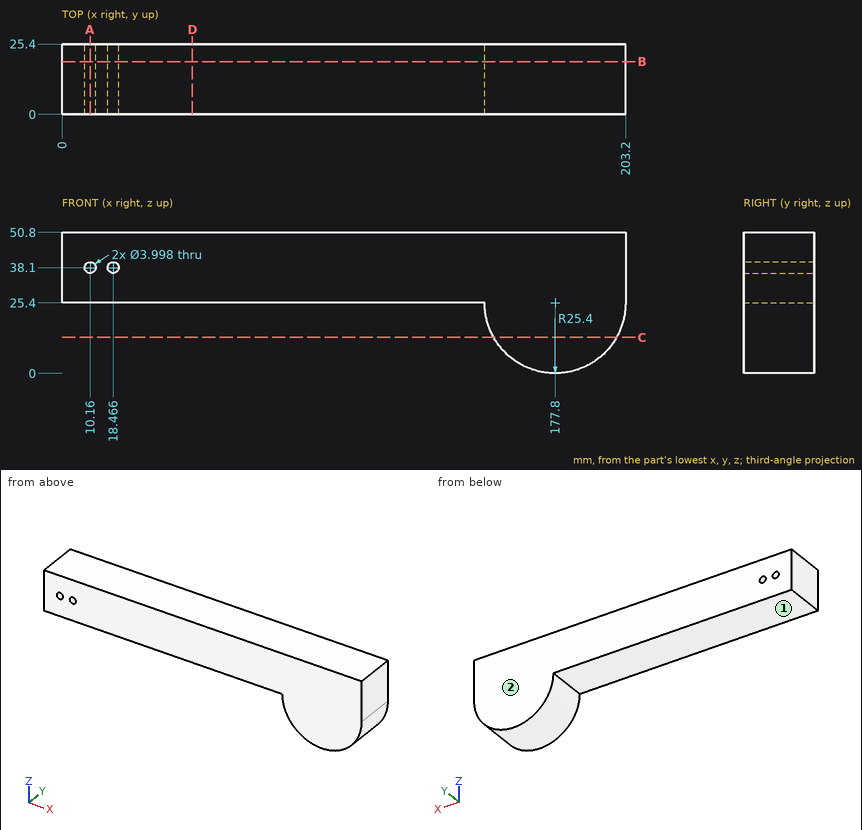
Study the drawing (mm; zero at the part's minimum x, y, z) and answer. A direction names the side the tool comes from. Give positions to 0.01 mm unless a question says otherwise; leave off trailing zeros. Write each loop counter-clockwise with the first axis right and the second up, starting at its lowest first coordinate (ties: lowest second). Pieces come first, ordered by that corner, then holes. Notation, with made-up numbers: (-34.5, -19) - (0.5, -19) arc R20 ccw to (0.5, -9) - close; hole circle Ø3 at (74.5, -16.5). An arc over 180 degrees is marked (long way). One line per question, with ' | ' between items. Start each with the question number.
1. Section D-D, the plane x = 47 is taken. Determine the outline of the cut face in (y, z).
2. Given P1, Ø1, axis at y = 6.5, z = 12.5, coming from the -X side; P2, Ø1, axis at y = 14.5, z = 23.5, coming from the -X side, each flat-ended and moving along its own axis, determine where each tip first touches the part or whether it passes through.
3. Straight lines are drawn through the part: line 1 (X direction, y = 20.25, z = 38.1) (1 decimal); line 2 (X direction, y = 16.25, z = 37) (1 decimal); line 3 (Z direction, x = 45.5, y = 2.25). For each, find the intervals that lie inside material, in ascending order.
4. Section C-C, the plane z = 13 is taken. Determine the outline of the cut face in (x, y).
5. Section A-A, the plane x = 10.16 is taken. Determine the outline of the cut face in (y, z).
6. For the marked faces 1 and 2, determine the directions among +Z, -Z, +X, -X, +Y, -Y from which every point of the face is accessible in a straight line to the end or side of a thin tool.
7. Section B-B, the plane y = 19 is taken. Determine the outline of the cut face in (x, z).
Result:
1) outline: (0, 25.4) - (25.4, 25.4) - (25.4, 50.8) - (0, 50.8) - close
2) P1: stops at x = 155.63 | P2: stops at x = 152.44
3) line 1: x = 0 to 8.2, 12.2 to 16.5, 20.5 to 203.2 | line 2: x = 0 to 8.5, 11.8 to 16.8, 20.1 to 203.2 | line 3: z = 25.4 to 50.8
4) outline: (155.63, 0) - (199.97, 0) - (199.97, 25.4) - (155.63, 25.4) - close
5) outline: (0, 25.4) - (25.4, 25.4) - (25.4, 36.1) - (0, 36.1) - close; (0, 40.1) - (25.4, 40.1) - (25.4, 50.8) - (0, 50.8) - close
6) face 1: -Z, -X, +Y, -Y | face 2: +Z, -Z, +X, -X, +Y
7) outline: (0, 25.4) - (152.4, 25.4) arc R25.4 ccw to (203.2, 25.4) - (203.2, 50.8) - (0, 50.8) - close; hole circle Ø4 at (10.16, 38.1); hole circle Ø4 at (18.47, 38.1)
